Source: CAD feature listing. Evaluate the final solid. Frame: model axes, mm. A direction names the side the tool comes from. Round coordinates to 2 decimals unless told otherwise and drop trailing zeros. Order: outer loops, then holes, each group sorted by start corner. A loop starts at its lowest first (then second) coordinate and runs counter-clockwise, first axis right, second up. Notation, with made-up numbers: (74.25, 35) - (131.25, 35) arc R33 ccw to (131.25, 69) - close; hole circle Ø8 at (-2, 2.25). An arc over 180 degrees is marked (long way). Use one line per item in the form item = value. Start each with the question number.
Q1. Draft query along X for faces 1 (the flat face through (0, 4, -34)), 2 (the flat face through (-6.6, 1, -34)), 3 (the flat face through (-16.55, 2, -34)). Return one class per face: released by +X, released by -X, zero draft, split by the parting line, or undercut.
Q2. Cut plane B-B, the plane x = -3.5. Return the cut outline in (y, z).
Q3. Set-up query: faces 4 (the flat face through (6.6, 1, -34)), 5 (the flat face through (-0.2, 2.4, -49)). Return all of +Z, -Z, +X, -X, +Y, -Y with unobstructed straight access to the full face (end or side cutting, diameter ignored); none if empty.
Q4. Ray query, line 1 (X direction, y = 1.6, z = -30.5); line 2 (X direction, y = 0.45, z = -46); line 3 (X direction, y = 3.6, z = -20). Return the intervals inside material, ascending. Write a range as [from, to].
Q5. Cut plane A-A, the plane z = -37.5. Return the cut outline in (x, y).
Q6. Pin query (flat end, axial travel): pin 1 Ø1.7 at (y, z) = (1, -34) entering from +X; pin 2 Ø4 at (x, z) = (3, -41) entering from -Y. Return the tip coordinate at first contact, or that it passes through.
from build123d import *

# Parameters (mm, degrees)
SKETCH1_W             = 3
SKETCH1_H             = 49
BOSS_EXTRUDE1_DEPTH   = 10
BOSS_EXTRUDE1_2_DEPTH = 10
BOSS_EXTRUDE2_START   = -10
SKETCH2_W             = 33.1
SKETCH2_H             = 30
BOSS_EXTRUDE2_DEPTH   = 4
CUT_EXTRUDE1_START    = -10
SKETCH3_W             = 13.2
SKETCH3_H             = 30
CUT_EXTRUDE1_DEPTH    = 2
CUT_EXTRUDE2_START    = -3
CUT_EXTRUDE2_DEPTH    = 2.5
CUT_EXTRUDE3_START    = -36.1
SKETCH6_R             = 1.6
CUT_EXTRUDE3_DEPTH    = 2.5
CUT_EXTRUDE4_START    = -3.4
CUT_EXTRUDE4_DEPTH    = 3.2
CUT_EXTRUDE6_DEPTH    = 54.695460702


with BuildPart() as part:
    # Sketch1 → Boss-Extrude1 (new body)
    with BuildSketch(Plane(origin=(0, 0, 0), x_dir=(1, 0, 0), z_dir=(0, 1, 0))):
        with Locations((-18.05, 24.5)):
            Rectangle(SKETCH1_W, SKETCH1_H)
    extrude(amount=BOSS_EXTRUDE1_DEPTH)



with BuildPart() as body_2:
    # Sketch1 → Boss-Extrude1 2 (new body)
    with BuildSketch(Plane(origin=(0, 0, 0), x_dir=(1, 0, 0), z_dir=(0, 1, 0))):
        with Locations((18.05, 24.5)):
            Rectangle(SKETCH1_W, SKETCH1_H)
    extrude(amount=BOSS_EXTRUDE1_2_DEPTH)


with BuildPart() as part_1:
    add(part.part)

    add(body_2.part)  # Boss-Extrude2 merges body 2
    # Sketch2 → Boss-Extrude2 (add)
    with BuildSketch(Plane(origin=(0, 10, 0), x_dir=(1, 0, 0), z_dir=(0, 1, 0)).offset(BOSS_EXTRUDE2_START)):
        with Locations((0, 34)):
            Rectangle(SKETCH2_W, SKETCH2_H)
    extrude(amount=BOSS_EXTRUDE2_DEPTH)

    # Sketch3 → Cut-Extrude1 (cut)
    with BuildSketch(Plane(origin=(0, 10, 0), x_dir=(1, 0, 0), z_dir=(0, 1, 0)).offset(CUT_EXTRUDE1_START)):
        with Locations((0, 34)):
            Rectangle(SKETCH3_W, SKETCH3_H)
    extrude(amount=CUT_EXTRUDE1_DEPTH, mode=Mode.SUBTRACT)

    # Sketch5 → Cut-Extrude2 (cut)
    with BuildSketch(Plane.ZY.offset(19.55).offset(CUT_EXTRUDE2_START)):
        with BuildLine():
            Line((-4.75, 7.236067977), (-4.854831539, 6.824677172))
            ThreePointArc((-4.854831539, 6.824677172), (-4.891407754, 6.769616655), (-4.954343768, 6.74940433))
            ThreePointArc((-4.954343768, 6.74940433), (-5, 6.75), (-5.045656232, 6.74940433))
            ThreePointArc((-5.045656232, 6.74940433), (-5.108592246, 6.769616655), (-5.145168461, 6.824677172))
            Line((-5.145168461, 6.824677172), (-5.25, 7.236067977))
            ThreePointArc((-5.25, 7.236067977), (-5.3907084, 7.215817444), (-5.529857135, 7.186721614))
            Line((-5.529857135, 7.186721614), (-5.487662617, 6.764286212))
            ThreePointArc((-5.487662617, 6.764286212), (-5.503201209, 6.700036448), (-5.555428696, 6.65951769))
            ThreePointArc((-5.555428696, 6.65951769), (-5.598535251, 6.644462086), (-5.641234343, 6.628286988))
            ThreePointArc((-5.641234343, 6.628286988), (-5.707287874, 6.625754976), (-5.760490079, 6.664985136))
            Line((-5.760490079, 6.664985136), (-5.999703445, 7.015711542))
            ThreePointArc((-5.999703445, 7.015711542), (-6.125, 6.948557159), (-6.24580568, 6.873624351))
            Line((-6.24580568, 6.873624351), (-6.061674385, 6.491096296))
            ThreePointArc((-6.061674385, 6.491096296), (-6.054301173, 6.425406755), (-6.089520725, 6.369468725))
            ThreePointArc((-6.089520725, 6.369468725), (-6.124878317, 6.340577775), (-6.15947013, 6.310774205))
            ThreePointArc((-6.15947013, 6.310774205), (-6.220674146, 6.285803254), (-6.28408537, 6.30447132))
            Line((-6.28408537, 6.30447132), (-6.628827901, 6.552230546))
            ThreePointArc((-6.628827901, 6.552230546), (-6.723599997, 6.446272122), (-6.811491673, 6.33454034))
            Line((-6.811491673, 6.33454034), (-6.507632554, 6.038058161))
            ThreePointArc((-6.507632554, 6.038058161), (-6.478236855, 5.978851971), (-6.492200475, 5.914241621))
            ThreePointArc((-6.492200475, 5.914241621), (-6.515544457, 5.875), (-6.537856707, 5.835162708))
            ThreePointArc((-6.537856707, 5.835162708), (-6.586829101, 5.790764683), (-6.652801015, 5.786619011))
            Line((-6.652801015, 5.786619011), (-7.061491673, 5.901527638))
            ThreePointArc((-7.061491673, 5.901527638), (-7.114308397, 5.769545322), (-7.158685036, 5.634491068))
            Line((-7.158685036, 5.634491068), (-6.771747987, 5.459814891))
            ThreePointArc((-6.771747987, 5.459814891), (-6.723875356, 5.414233193), (-6.714898826, 5.348743485))
            ThreePointArc((-6.714898826, 5.348743485), (-6.723413568, 5.303884311), (-6.730755068, 5.258818263))
            ThreePointArc((-6.730755068, 5.258818263), (-6.761589047, 5.200348221), (-6.822164464, 5.17388884))
            Line((-6.822164464, 5.17388884), (-7.245509125, 5.142087191))
            ThreePointArc((-7.245509125, 5.142087191), (-7.25, 5), (-7.245509125, 4.857912809))
            Line((-7.245509125, 4.857912809), (-6.822164464, 4.82611116))
            ThreePointArc((-6.822164464, 4.82611116), (-6.761589047, 4.799651779), (-6.730755068, 4.741181737))
            ThreePointArc((-6.730755068, 4.741181737), (-6.723413568, 4.696115689), (-6.714898826, 4.651256515))
            ThreePointArc((-6.714898826, 4.651256515), (-6.723875356, 4.585766807), (-6.771747987, 4.540185109))
            Line((-6.771747987, 4.540185109), (-7.158685036, 4.365508932))
            ThreePointArc((-7.158685036, 4.365508932), (-7.114308397, 4.230454678), (-7.061491673, 4.098472362))
            Line((-7.061491673, 4.098472362), (-6.652801015, 4.213380989))
            ThreePointArc((-6.652801015, 4.213380989), (-6.586829101, 4.209235317), (-6.537856707, 4.164837292))
            ThreePointArc((-6.537856707, 4.164837292), (-6.515544457, 4.125), (-6.492200475, 4.085758379))
            ThreePointArc((-6.492200475, 4.085758379), (-6.478236855, 4.021148029), (-6.507632554, 3.961941839))
            Line((-6.507632554, 3.961941839), (-6.811491673, 3.66545966))
            ThreePointArc((-6.811491673, 3.66545966), (-6.723599997, 3.553727878), (-6.628827901, 3.447769454))
            Line((-6.628827901, 3.447769454), (-6.28408537, 3.69552868))
            ThreePointArc((-6.28408537, 3.69552868), (-6.220674146, 3.714196746), (-6.15947013, 3.689225795))
            ThreePointArc((-6.15947013, 3.689225795), (-6.124878317, 3.659422225), (-6.089520725, 3.630531275))
            ThreePointArc((-6.089520725, 3.630531275), (-6.054301173, 3.574593245), (-6.061674385, 3.508903704))
            Line((-6.061674385, 3.508903704), (-6.24580568, 3.126375649))
            ThreePointArc((-6.24580568, 3.126375649), (-6.125, 3.051442841), (-5.999703445, 2.984288458))
            Line((-5.999703445, 2.984288458), (-5.760490079, 3.335014864))
            ThreePointArc((-5.760490079, 3.335014864), (-5.707287874, 3.374245024), (-5.641234343, 3.371713012))
            ThreePointArc((-5.641234343, 3.371713012), (-5.598535251, 3.355537914), (-5.555428696, 3.34048231))
            ThreePointArc((-5.555428696, 3.34048231), (-5.503201209, 3.299963552), (-5.487662617, 3.235713788))
            Line((-5.487662617, 3.235713788), (-5.529857135, 2.813278386))
            ThreePointArc((-5.529857135, 2.813278386), (-5.3907084, 2.784182556), (-5.25, 2.763932023))
            Line((-5.25, 2.763932023), (-5.145168461, 3.175322828))
            ThreePointArc((-5.145168461, 3.175322828), (-5.108592246, 3.230383345), (-5.045656232, 3.25059567))
            ThreePointArc((-5.045656232, 3.25059567), (-5, 3.25), (-4.954343768, 3.25059567))
            ThreePointArc((-4.954343768, 3.25059567), (-4.891407754, 3.230383345), (-4.854831539, 3.175322828))
            Line((-4.854831539, 3.175322828), (-4.75, 2.763932023))
            ThreePointArc((-4.75, 2.763932023), (-4.6092916, 2.784182556), (-4.470142865, 2.813278386))
            Line((-4.470142865, 2.813278386), (-4.512337383, 3.235713788))
            ThreePointArc((-4.512337383, 3.235713788), (-4.496798791, 3.299963552), (-4.444571304, 3.34048231))
            ThreePointArc((-4.444571304, 3.34048231), (-4.401464749, 3.355537914), (-4.358765657, 3.371713012))
            ThreePointArc((-4.358765657, 3.371713012), (-4.292712126, 3.374245024), (-4.239509921, 3.335014864))
            Line((-4.239509921, 3.335014864), (-4.000296555, 2.984288458))
            ThreePointArc((-4.000296555, 2.984288458), (-3.875, 3.051442841), (-3.75419432, 3.126375649))
            Line((-3.75419432, 3.126375649), (-3.938325615, 3.508903704))
            ThreePointArc((-3.938325615, 3.508903704), (-3.945698827, 3.574593245), (-3.910479275, 3.630531275))
            ThreePointArc((-3.910479275, 3.630531275), (-3.875121683, 3.659422225), (-3.84052987, 3.689225795))
            ThreePointArc((-3.84052987, 3.689225795), (-3.779325854, 3.714196746), (-3.71591463, 3.69552868))
            Line((-3.71591463, 3.69552868), (-3.371172099, 3.447769454))
            ThreePointArc((-3.371172099, 3.447769454), (-3.276400003, 3.553727878), (-3.188508327, 3.66545966))
            Line((-3.188508327, 3.66545966), (-3.492367446, 3.961941839))
            ThreePointArc((-3.492367446, 3.961941839), (-3.521763145, 4.021148029), (-3.507799525, 4.085758379))
            ThreePointArc((-3.507799525, 4.085758379), (-3.484455543, 4.125), (-3.462143293, 4.164837292))
            ThreePointArc((-3.462143293, 4.164837292), (-3.413170899, 4.209235317), (-3.347198985, 4.213380989))
            Line((-3.347198985, 4.213380989), (-2.938508327, 4.098472362))
            ThreePointArc((-2.938508327, 4.098472362), (-2.885691603, 4.230454678), (-2.841314964, 4.365508932))
            Line((-2.841314964, 4.365508932), (-3.228252013, 4.540185109))
            ThreePointArc((-3.228252013, 4.540185109), (-3.276124644, 4.585766807), (-3.285101174, 4.651256515))
            ThreePointArc((-3.285101174, 4.651256515), (-3.276586432, 4.696115689), (-3.269244932, 4.741181737))
            ThreePointArc((-3.269244932, 4.741181737), (-3.238410953, 4.799651779), (-3.177835536, 4.82611116))
            Line((-3.177835536, 4.82611116), (-2.754490875, 4.857912809))
            ThreePointArc((-2.754490875, 4.857912809), (-2.75, 5), (-2.754490875, 5.142087191))
            Line((-2.754490875, 5.142087191), (-3.177835536, 5.17388884))
            ThreePointArc((-3.177835536, 5.17388884), (-3.238410953, 5.200348221), (-3.269244932, 5.258818263))
            ThreePointArc((-3.269244932, 5.258818263), (-3.276586432, 5.303884311), (-3.285101174, 5.348743485))
            ThreePointArc((-3.285101174, 5.348743485), (-3.276124644, 5.414233193), (-3.228252013, 5.459814891))
            Line((-3.228252013, 5.459814891), (-2.841314964, 5.634491068))
            ThreePointArc((-2.841314964, 5.634491068), (-2.885691603, 5.769545322), (-2.938508327, 5.901527638))
            Line((-2.938508327, 5.901527638), (-3.347198985, 5.786619011))
            ThreePointArc((-3.347198985, 5.786619011), (-3.413170899, 5.790764683), (-3.462143293, 5.835162708))
            ThreePointArc((-3.462143293, 5.835162708), (-3.484455543, 5.875), (-3.507799525, 5.914241621))
            ThreePointArc((-3.507799525, 5.914241621), (-3.521763145, 5.978851971), (-3.492367446, 6.038058161))
            Line((-3.492367446, 6.038058161), (-3.188508327, 6.33454034))
            ThreePointArc((-3.188508327, 6.33454034), (-3.276400003, 6.446272122), (-3.371172099, 6.552230546))
            Line((-3.371172099, 6.552230546), (-3.71591463, 6.30447132))
            ThreePointArc((-3.71591463, 6.30447132), (-3.779325854, 6.285803254), (-3.84052987, 6.310774205))
            ThreePointArc((-3.84052987, 6.310774205), (-3.875121683, 6.340577775), (-3.910479275, 6.369468725))
            ThreePointArc((-3.910479275, 6.369468725), (-3.945698827, 6.425406755), (-3.938325615, 6.491096296))
            Line((-3.938325615, 6.491096296), (-3.75419432, 6.873624351))
            ThreePointArc((-3.75419432, 6.873624351), (-3.875, 6.948557159), (-4.000296555, 7.015711542))
            Line((-4.000296555, 7.015711542), (-4.239509921, 6.664985136))
            ThreePointArc((-4.239509921, 6.664985136), (-4.292712126, 6.625754976), (-4.358765657, 6.628286988))
            ThreePointArc((-4.358765657, 6.628286988), (-4.401464749, 6.644462086), (-4.444571304, 6.65951769))
            ThreePointArc((-4.444571304, 6.65951769), (-4.496798791, 6.700036448), (-4.512337383, 6.764286212))
            Line((-4.512337383, 6.764286212), (-4.470142865, 7.186721614))
            ThreePointArc((-4.470142865, 7.186721614), (-4.6092916, 7.215817444), (-4.75, 7.236067977))
        make_face()
    extrude(amount=CUT_EXTRUDE2_DEPTH, mode=Mode.SUBTRACT)

    # Sketch6 → Cut-Extrude3 (cut)
    with BuildSketch(Plane.ZY.offset(19.55).offset(CUT_EXTRUDE3_START)):
        with Locations(Location((-5, 5, 0), (0, 0, 180))):
            Circle(SKETCH6_R)
    extrude(amount=-CUT_EXTRUDE3_DEPTH, mode=Mode.SUBTRACT)

    # Sketch9 → Cut-Extrude4 (cut)
    with BuildSketch(Plane(origin=(0, 10, 0), x_dir=(1, 0, 0), z_dir=(0, 1, 0)).offset(CUT_EXTRUDE4_START)):
        Polygon((16.55, 5), (17.55, 5), (19.05, 0), (16.55, 0), align=None)
    extrude(amount=-CUT_EXTRUDE4_DEPTH, mode=Mode.SUBTRACT)

    # Sketch10 → Cut-Extrude6 (cut, through all)
    with BuildSketch(Plane(origin=(0, 0, -49), x_dir=(-1, 0, 0), z_dir=(0, 0, -1))):
        Polygon((-15.644123368, 2.927582789), (-16.55, 3.35), (-16.55, 1.05), (-15.534888499, 1.523354267), (-15.534888499, -2.347783868), (-19.962773438, -2.347783868), (-19.962773438, 10.874284902), (-15.644123368, 10.874284902), align=None)
        Polygon((19.962773438, 10.874284902), (15.644123368, 10.874284902), (15.644123368, 2.927582789), (16.55, 3.35), (16.55, 1.05), (15.534888499, 1.523354267), (15.534888499, -2.347783868), (19.962773438, -2.347783868), align=None)
    extrude(amount=-CUT_EXTRUDE6_DEPTH, mode=Mode.SUBTRACT)


solid = part_1.part
Completed:
q1.face_1 = zero draft
q1.face_2 = undercut
q1.face_3 = released by -X
q2.outline = (2, -49) - (4, -49) - (4, -19) - (2, -19) - close
q3.face_4 = +Z, -Z, -Y
q3.face_5 = -Z, +X, -X, +Y, -Y
q4.line_1 = [-16.55, -6.6], [6.6, 16.55]
q4.line_2 = [-15.53, -6.6], [6.6, 15.53]
q4.line_3 = [-15.64, 15.64]
q5.outline = (-16.55, 1.05) - (-15.53, 1.52) - (-15.53, 0) - (-6.6, 0) - (-6.6, 2) - (6.6, 2) - (6.6, 0) - (15.53, 0) - (15.53, 1.52) - (16.55, 1.05) - (16.55, 3.35) - (15.64, 2.93) - (15.64, 4) - (-15.64, 4) - (-15.64, 2.93) - (-16.55, 3.35) - close
q6.pin_1 = 16.55
q6.pin_2 = 2
